```python
from build123d import *

# Parameters (mm, degrees)
SKETCH1_W           = 56
SKETCH1_H           = 56
SKETCH1_R           = 2.45
BOSS_EXTRUDE1_DEPTH = 10
SKETCH2_R           = 1.45
CUT_EXTRUDE1_DEPTH  = 80.824808174
FILLET1_R           = 20


with BuildPart() as part:
    # Sketch1 → Boss-Extrude1 (new body)
    with BuildSketch(Plane(origin=(0, 0, 0), x_dir=(1, 0, 0), z_dir=(0, 1, 0))):
        with Locations((28, 28)):
            Rectangle(SKETCH1_W, SKETCH1_H)
        with Locations(Location((28, 28, 0), (0, 0, 270))):
            Circle(SKETCH1_R, mode=Mode.SUBTRACT)
        with Locations(Location((12, 44, 0), (0, 0, 270))):
            Circle(SKETCH1_R, mode=Mode.SUBTRACT)
        with Locations(Location((44, 44, 0), (0, 0, 270))):
            Circle(SKETCH1_R, mode=Mode.SUBTRACT)
        with Locations(Location((44, 12, 0), (0, 0, 270))):
            Circle(SKETCH1_R, mode=Mode.SUBTRACT)
        with Locations(Location((12, 12, 0), (0, 0, 270))):
            Circle(SKETCH1_R, mode=Mode.SUBTRACT)
    extrude(amount=BOSS_EXTRUDE1_DEPTH)

    # Sketch2 → Cut-Extrude1 (cut, through all)
    with BuildSketch(Plane.XY):
        with Locations((2.5, 2.5)):
            Circle(SKETCH2_R)
    extrude(amount=-CUT_EXTRUDE1_DEPTH, mode=Mode.SUBTRACT)

    # Fillet1
    fillet1_edges = [part.edges().sort_by_distance(p)[0] for p in [
        (56, 5, -56),
        (56, 5, 0),
    ]]
    fillet(fillet1_edges, radius=FILLET1_R)


solid = part.part
```
For this review, take the finished solid that the model builds, in its own axes (mm). Round coordinates to 2 decimals unless told otherwise and drop trailing zeros. Write each loop counter-clockwise with the first axis right and the second up, starting at its lowest first coordinate (ties: lowest second). Pieces come first, ordered by that corner, then holes. Notation, with made-up numbers: (68, 72.25) -> (72, 72.25) arc R27 ccw to (72, 100.25) -> close; hole circle Ø11 at (-19, 56.5). An arc over 180 degrees is marked (long way). One line per question, with ' | ' between items. Start each with the question number.
1) Add section D-D (x = 12). Write out the cut boundary in (y, z).
2) Mouldability with a two-part tool opening along Z and no side actions: class faces 1 (the flat face through (18, 5, -56)), 2 (the cylindrical face through (46.43, 4.93, -12.32)), 3 (the flat face through (21, 0, -28)) as +Z half, -Z half, draft (parallel to the pull), parting line (faces both ways), or undercut.
3) Wall thickness on line 1 along Z through (x, y) = (45, 5.75); line 2 along X through (y, z) = (4, -12); line 3 along Y through (x, z) = (2.5, -14.5): over which ranges is each line inside the solid? List them lowest first.
4) Add section A-A (z = -28). Write out the cut boundary in (x, y).
5) For pin 1 Ø3 at (x, z) = (12, -44) entering from -Y; pin 2 Ø1 at (x, y) = (50.5, 7) entering from -Z; pin 3 Ø2 at (x, y) = (46.5, 6.5) entering from +Z; pin 4 Ø5.5 at (x, z) = (44, -44) entering from -Y, all flat-tipped, find the tip position at first contact; note any pin that passes through.
6) Add section B-B (y = 2.5). Write out the cut boundary in (x, z).
7) Add section C-C (x = 2.5). Write out the cut boundary in (y, z), and give its area (3 significant figures).
Reported:
1) outline: (0, -56) -> (10, -56) -> (10, -46.45) -> (0, -46.45) -> close; (0, -41.55) -> (10, -41.55) -> (10, -14.45) -> (0, -14.45) -> close; (0, -9.55) -> (10, -9.55) -> (10, 0) -> (0, 0) -> close
2) face 1: -Z half | face 2: undercut | face 3: draft
3) line 1: z = -53.86 to -46.24, -41.76 to -14.24, -9.76 to -2.14 | line 2: x = 0 to 9.55, 14.45 to 41.55, 46.45 to 54.33 | line 3: y = 0 to 1.05, 3.95 to 10
4) outline: (0, 0) -> (25.55, 0) -> (25.55, 10) -> (0, 10) -> close; (30.45, 0) -> (56, 0) -> (56, 10) -> (30.45, 10) -> close; hole circle Ø2.9 at (2.5, 2.5)
5) pin 1: passes through | pin 2: stops at z = -50.28 | pin 3: stops at z = -2.4 | pin 4: stops at y = 0
6) outline: (0, -56) -> (1.05, -56) -> (1.05, 0) -> (0, 0) -> close; (3.95, -56) -> (36, -56) arc R20 ccw to (56, -36) -> (56, -20) arc R20 ccw to (36, 0) -> (3.95, 0) -> close; hole circle Ø4.9 at (12, -44); hole circle Ø4.9 at (12, -12); hole circle Ø4.9 at (28, -28); hole circle Ø4.9 at (44, -44); hole circle Ø4.9 at (44, -12)
7) outline: (0, -56) -> (1.05, -56) -> (1.05, 0) -> (0, 0) -> close; (3.95, -56) -> (10, -56) -> (10, 0) -> (3.95, 0) -> close | area: 398 mm²
